Answer from the drawing. Dimensions are ordinates in mm from the lowest x, y and z of the part. Give positions to 0.01 mm unless a question says otherwise; leave off trailing zeros. Write each loop counter-clockwise with the first axis right and the second up, starting at its lowest first coordinate (ties: lowest second). Pieces come first, ordered by that corner, then holes. Notation, with made-up numbers: (40.5, -35) -> (47.5, -35) arc R14 cw to (47.5, -8) -> close; hole circle Ø6 at (-26.5, 26). An arc over 180 degrees is marked (long way). Write item = value, one per line.
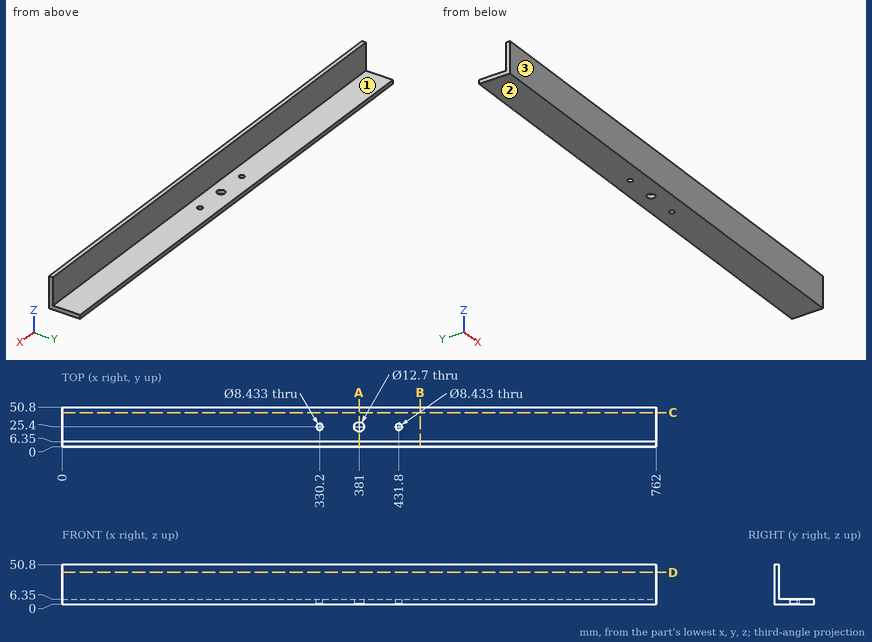
(1) The part is cut by section B-B on x = 459. Determine the outline of the cut face in (y, z).
Checks:
outline = (0, 0) -> (50.8, 0) -> (50.8, 6.35) -> (6.35, 6.35) -> (6.35, 50.8) -> (0, 50.8) -> close
(2) Consider L1, parallel to X at y = 25.4, z = 2.5; L2, parallel to Y at x = 330, z = 2; L3, parallel to Z at x = 628.5, y = 24. Determine where each line is inside the solid, lowest interval first.
Checks:
L1 = 0 to 325.98, 334.42 to 374.65, 387.35 to 427.58, 436.02 to 762
L2 = 0 to 21.19, 29.61 to 50.8
L3 = 0 to 6.35
(3) For a pull along Z with two mould halves and no side action, classify the marked faces 1, 2 and 3 as released by +Z, released by -Z, zero draft, split by the parting line, or undercut.
Checks:
face_1 = released by +Z
face_2 = released by -Z
face_3 = zero draft
(4) Given P1, Ø22, axis at x = 344.5, z = 35.5, coming from the +Y side; P2, Ø11, axis at x = 431.8, y = 25.4, coming from the +Z side, each flat-ended and moving along its own axis, determine where each tip first touches the part or whether it passes through.
Checks:
P1 = 6.35
P2 = 6.35
(5) The part is cut by section A-A on x = 381. Determine the outline of the cut face in (y, z), plus the area to 3 significant figures.
Checks:
outline = (0, 0) -> (19.05, 0) -> (19.05, 6.35) -> (6.35, 6.35) -> (6.35, 50.8) -> (0, 50.8) -> close; (31.75, 0) -> (50.8, 0) -> (50.8, 6.35) -> (31.75, 6.35) -> close
area = 524 mm²
(6) The part is cut by section C-C on y = 43.5. Determine the outline of the cut face in (x, z), plus the area to 3 significant figures.
Checks:
outline = (0, 0) -> (762, 0) -> (762, 6.35) -> (0, 6.35) -> close
area = 4,840 mm²
